Build history of the part. All positions in model axes, mm. A direction names the side the tool comes from. Coordinates: 2 decimals unless noted, no trailing zeros. Write each loop counter-clockwise with the first axis right and the second up, starting at its lowest first coordinate (ties: lowest second). Pieces come first, ordered by that corner, then holes.
```python
from build123d import *

# Parameters (mm, degrees)
F0_W     = 101.6
F0_H     = 101.6
F1_DEPTH = 101.6
F2_R     = 25.4
F3_DEPTH = 101.6
F6_W     = 50.8
F6_H     = 50.8
F7_DEPTH = 101.6
F8_R     = 5.08


with BuildPart() as f1:
    # F0 (on Top) → F1 (new body)
    with BuildSketch(Plane.XY):
        Rectangle(F0_W, F0_H)
    extrude(amount=F1_DEPTH)

    # F2 (on face) → F3 (join)
    with BuildSketch(Plane.XY.offset(101.6)):
        Circle(F2_R)
    extrude(amount=F3_DEPTH)

    # F4 (on face) → F5 (revolve)
    with BuildSketch(Plane.XY.offset(203.2)):
        with BuildLine():
            Line((0, -25.4), (0, -38.1))
            ThreePointArc((0, -38.1), (38.1, 0), (0, 38.1))
            Line((0, 38.1), (0, 25.4))
            ThreePointArc((0, 25.4), (17.9605122421, 17.9605122421), (25.4, 0))
            ThreePointArc((25.4, 0), (17.9605122421, -17.9605122421), (0, -25.4))
        make_face()
        with BuildLine():
            Line((0, 25.4), (0, -25.4))
            ThreePointArc((0, -25.4), (17.9605122421, -17.9605122421), (25.4, 0))
            ThreePointArc((25.4, 0), (17.9605122421, 17.9605122421), (0, 25.4))
        make_face()
    revolve(axis=Axis((0, 0, 203.2), (0, -1, 0)))

    # F6 (on face) → F7 (cut)
    with BuildSketch(Plane.XZ.offset(50.8)):
        with Locations((0, 50.8)):
            Rectangle(F6_W, F6_H)
    extrude(amount=-F7_DEPTH, mode=Mode.SUBTRACT)

    # F8
    f8_edges = [f1.edges().sort_by_distance(p)[0] for p in [
        (-25.4, 0, 101.6),
        (25.4, 0, 138.200968),
        (-25.4, 0, 174.801937),
        (50.8, 0, 101.6),
        (0, -50.8, 101.6),
        (0, 50.8, 101.6),
        (-50.8, 0, 101.6),
        (50.8, -50.8, 50.8),
        (50.8, 50.8, 50.8),
        (50.8, 0, 0),
        (0, 50.8, 0),
        (-50.8, 0, 0),
        (0, -50.8, 0),
    ]]
    fillet(f8_edges, radius=F8_R)


solid = f1.part
```
1. Saw through at D-D on z = 186.5. List the corners of the cut face in (x, y) (3 decimals), plus the area to 3 significant figures.
Computed values:
outline: circle Ø68.49 at (0, 0)
area: 3,680 mm2
2. 3-axis set-ups, long thin cutter, end or side, ignore diameter. For faces 1 (the face through (49.351, 0.64, 1.528)), 2 (the face through (-1, 31, 101.6)), 3 (the face through (25.4, -1, 50)): which of +Z, -Z, +X, -X, +Y, -Y reach the whole face in a straight line?
Computed values:
face 1: -Z, +X, +Y, -Y
face 2: none
face 3: +Y, -Y
3. Saw through at C-C on z = 152. List the corners of the cut face in (x, y), plus the area to 3 significant figures.
Computed values:
outline: circle Ø50.8 at (0, 0)
area: 2,030 mm2
4. Mould opens along X. For faces 4 (the face through (-25.4, -1, 50)), 5 (the face through (0, -1, 76.2)), 6 (the face through (-50.8, -1, 50)), 7 (the face through (-1.864, -49.272, 100.151)) say: +X half, -X half, draft (parallel to the pull), parting line (faces both ways), or undercut.
Computed values:
face 4: undercut
face 5: undercut
face 6: -X half
face 7: draft
5. Saw through at B-B on x = -43. List the corners of the cut face in (y, z), plus the area to 3 significant figures.
Computed values:
outline: (-50.8, 5.08) arc R5.08 ccw to (-45.72, 0) - (45.72, 0) arc R5.08 ccw to (50.8, 5.08) - (50.8, 96.52) arc R5.08 ccw to (45.72, 101.6) - (-45.72, 101.6) arc R5.08 ccw to (-50.8, 96.52) - close
area: 10,300 mm2
6. Saw through at A-A on z = 53. List the corners of the cut face in (x, y).
Computed values:
outline: (-50.8, -50.8) - (-25.4, -50.8) - (-25.4, 50.8) - (-50.8, 50.8) - close; (25.4, -50.8) - (45.72, -50.8) arc R5.08 ccw to (50.8, -45.72) - (50.8, 45.72) arc R5.08 ccw to (45.72, 50.8) - (25.4, 50.8) - close
7. Probe line 1 along Z through (x, y) = (-25, 42.5); line 2 along Z through (x, y) = (8.5, 32); line 3 along X through (y, z) = (-23, 74.5). List the from-to ranges inside material, lowest first.
Computed values:
line 1: z = 0 to 25.4, 76.2 to 101.6
line 2: z = 0 to 25.4, 76.2 to 101.6, 184.35 to 222.05
line 3: x = -50.8 to -25.4, 25.4 to 50.8
8. Flat gauge pins, fed straight in: pin 1 (8 mm diameter, centred on y = 27.5, z = 181, fed in from +X); pin 2 (1.5 mm diameter, centred on y = 4.5, z = 156.5, fed in from +X); pin 3 (2 mm diameter, centred on x = -16.5, y = 23.5, fed in from +Z). Where does each tip first touch, or does it go through?
Computed values:
pin 1: stops at x = 21.66
pin 2: stops at x = 25.12
pin 3: stops at z = 229.34
